Input: dimensioned drawing with shaded views. Units: mm. Origin: part minimum x, y, z. A direction names the side the tool comes from. Round coordinates to 2 decimals unless told otherwise and drop trailing zeros. Loops run counter-clockwise (first coordinate to the right, second up) from the corner with the lowest first, then second, coordinate; pieces in that order, holes last. Notation, with made-up numbers: (63.25, -18) - (72.25, -18) arc R16 ccw to (72.25, -5) - close; hole circle Ø5 at (-17.75, -38.75). An arc over 180 degrees is marked (long way). One line per question, with ' | ' between items. Start each with the question number.
1. Mould query, pull axis Y, two halves, no side actions, for the marked faces 3, 4 and 5. Classes: pulls with the +Y half, pulls with the -Y half, needs draft (parallel to the pull), parting line crosses it, or undercut.
2. Cut plane B-B (x = 41). Return loops of the section in (y, z).
3. Pin query (flat end, axial travel): pin 1 (8 mm diameter, centred on x = 31, z = 30.5, fed in from +Y); pin 2 (11.5 mm diameter, centred on x = 23, y = 37, fed in from +Z). Return the tip coordinate at first contact, or that it passes through.
4. Cut plane D-D (z = 15). Return loops of the section in (x, y) (1 decimal).
5. Access query for the marked faces 1 and 2. Directions: +Z, -Z, +X, -X, +Y, -Y. A direction counts if a zero-diameter tool reaches every point of the face in a straight line with its end or side. Return the directions, or none.
6. Cut plane C-C (y = 5.5). Return loops of the section in (x, z) (1 decimal), then the cut area to 3 significant figures.
7. Ray query, line 1 (Y direction, x = 40.5, z = 18.5); line 2 (X direction, y = 16, z = 53.5) (1 decimal); line 3 (Z direction, x = 34.5, y = 52.5). Return the intervals inside material, ascending.
8. Cut plane A-A (z = 36). Return loops of the section in (x, y) (1 decimal).
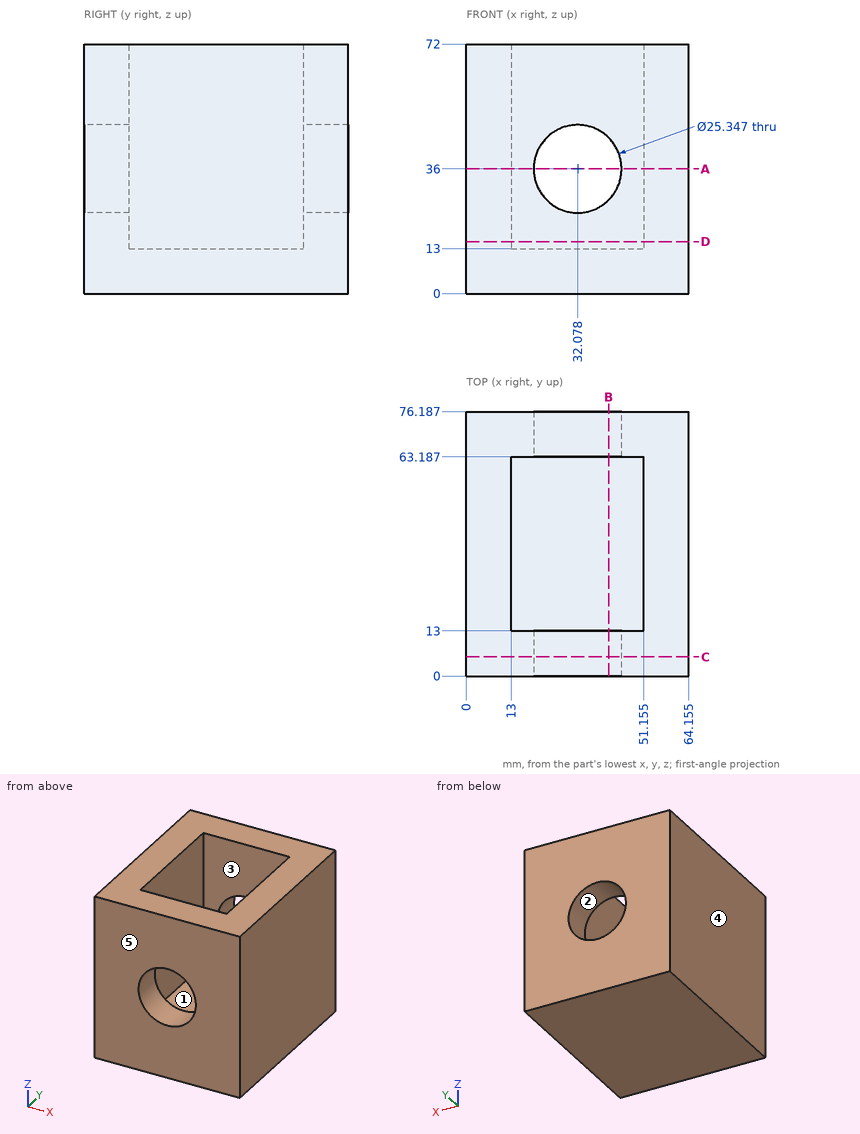
Answers follow:
1) face 3: undercut | face 4: needs draft | face 5: pulls with the -Y half
2) outline: (0, 0) - (76.19, 0) - (76.19, 27) - (63.19, 27) - (63.19, 13) - (13, 13) - (13, 27) - (0, 27) - close; (0, 45) - (13, 45) - (13, 72) - (0, 72) - close; (63.19, 45) - (76.19, 45) - (76.19, 72) - (63.19, 72) - close
3) pin 1: passes through | pin 2: stops at z = 13
4) outline: (0, 0) - (64.2, 0) - (64.2, 76.2) - (0, 76.2) - close; hole (13, 13) - (51.2, 13) - (51.2, 63.2) - (13, 63.2) - close
5) face 1: +Z | face 2: +Y, -Y
6) outline: (0, 0) - (64.2, 0) - (64.2, 72) - (0, 72) - close; hole circle Ø25.3 at (32.1, 36) | area: 4,110 mm2
7) line 1: y = 0 to 13, 63.19 to 76.19 | line 2: x = 0 to 13, 51.2 to 64.2 | line 3: z = 0 to 13
8) outline: (0, 0) - (19.4, 0) - (19.4, 13) - (13, 13) - (13, 63.2) - (19.4, 63.2) - (19.4, 76.2) - (0, 76.2) - close; (44.8, 0) - (64.2, 0) - (64.2, 76.2) - (44.8, 76.2) - (44.8, 63.2) - (51.2, 63.2) - (51.2, 13) - (44.8, 13) - close
